Drawing for the job (mm, zero at the part's lowest x, y, z). Give positions to 0.01 mm unless a question says otherwise; leave off trailing zeros. Order: outer loops, then holes, each group sorted by start corner. A loop starts at its lowest first (then second) coordinate and runs counter-clockwise, first axis right, second up. Notation, with made-up numbers: M -11,30.25 L 2,30.25 A27 cw 2,46.25 Z; hole C -17,-1 d3. An arc over 180 degrees is marked long. Answer as a JSON object with one key per item and string values.
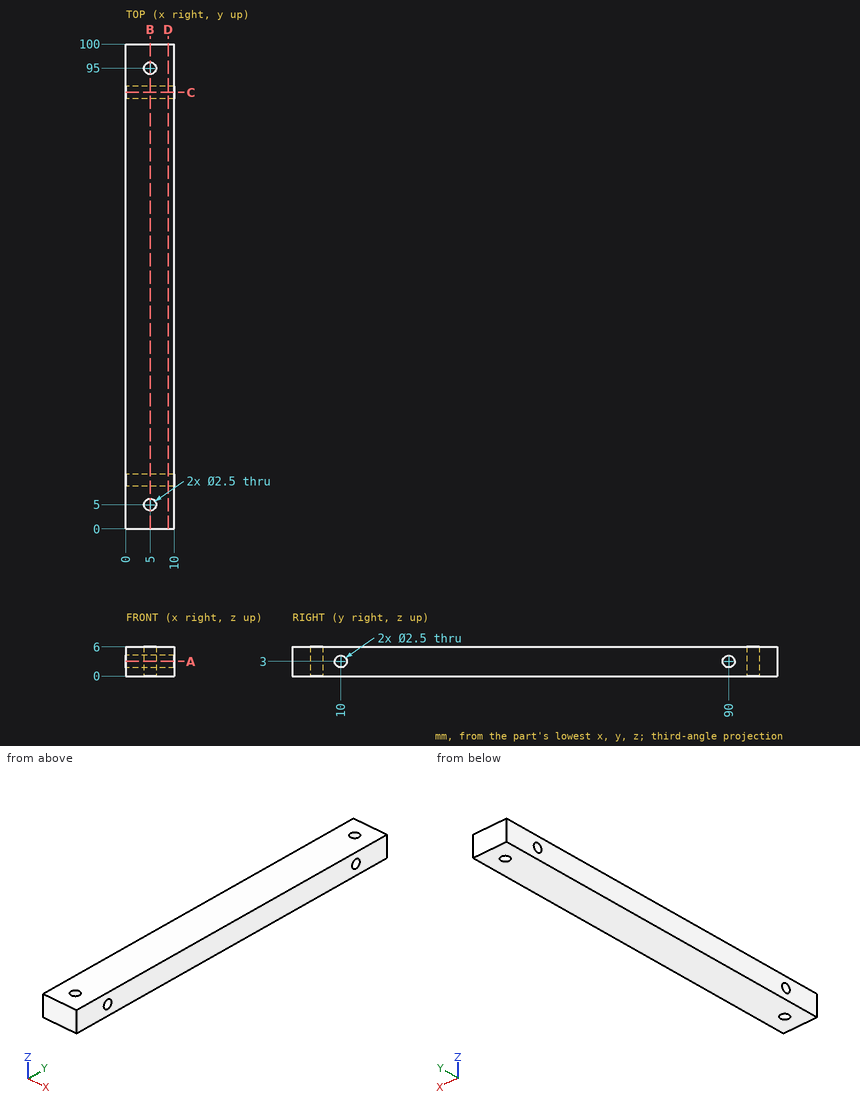
1. Cut at D-D on x = 8.75. Give the cut face in (y, z).
Worked answers:
{"outline": "M 0,0 L 100,0 L 100,6 L 0,6 Z; hole C 10,3 d2.5; hole C 90,3 d2.5"}
2. Probe line 1 along Y through (x, z) = (5, 1.7); line 2 along Y through (x, z) = (7, 3); line 3 along Y through (x, z) = (4.25, 3). List the from-to ranges inside material, lowest first.
Worked answers:
{"line 1": "y = 0 to 3.75, 6.25 to 93.75, 96.25 to 100", "line 2": "y = 0 to 8.75, 11.25 to 88.75, 91.25 to 100", "line 3": "y = 0 to 4, 6 to 8.75, 11.25 to 88.75, 91.25 to 94, 96 to 100"}
3. Cut at C-C on y = 90. Give the cut face in (x, z), plus the area to 3 significant figures.
Worked answers:
{"outline": "M 0,0 L 10,0 L 10,1.75 L 0,1.75 Z; M 0,4.25 L 10,4.25 L 10,6 L 0,6 Z", "area": "35.0 mm^2"}
4. Cut at A-A on z = 3. Give the cut face in (x, y), plus the area to 3 significant figures.
Worked answers:
{"outline": "M 0,0 L 10,0 L 10,8.75 L 0,8.75 Z; M 0,11.25 L 10,11.25 L 10,88.75 L 0,88.75 Z; M 0,91.25 L 10,91.25 L 10,100 L 0,100 Z; hole C 5,5 d2.5; hole C 5,95 d2.5", "area": "940 mm^2"}
5. Pin check, flat tips, straight feed: P1, Ø3, axis at y = 10, z = 3, coming from the +X side; P2, Ø2, axis at y = 90, z = 3, coming from the +X side. Stop position of each tip, or through.
Worked answers:
{"P1": "stops at x = 10", "P2": "passes through"}
6. Cut at B-B on x = 5. Give the cut face in (y, z), plus the area to 3 significant figures.
Worked answers:
{"outline": "M 0,0 L 3.75,0 L 3.75,6 L 0,6 Z; M 6.25,0 L 93.75,0 L 93.75,6 L 6.25,6 Z; M 96.25,0 L 100,0 L 100,6 L 96.25,6 Z; hole C 10,3 d2.5; hole C 90,3 d2.5", "area": "560 mm^2"}
